from build123d import *

# Parameters (mm, degrees)
F0_W     = 24
F0_H     = 63
F1_DEPTH = 12.5
F2_W     = 3.2
F2_H     = 55
F3_DEPTH = 4
F4_W     = 16
F4_H     = 3.2
F5_DEPTH = 4


with BuildPart() as f1:
    # F0 (on Top) → F1 (new body)
    with BuildSketch(Plane.XY):
        with Locations((12, 31.5)):
            Rectangle(F0_W, F0_H)
    extrude(amount=F1_DEPTH)

    # F2 (on face) → F3 (cut)
    with BuildSketch(Plane.XY.offset(12.5)):
        with Locations((7.15, 31.5)):
            Rectangle(F2_W, F2_H)
        with Locations((12.25, 31.5)):
            Rectangle(F2_W, F2_H)
        with Locations((17.35, 31.5)):
            Rectangle(F2_W, F2_H)
    extrude(amount=-F3_DEPTH, mode=Mode.SUBTRACT)

    # F4 (on face) → F5 (cut)
    with BuildSketch(Plane.XY.offset(12.5)):
        with Locations((12, 57.4)):
            Rectangle(F4_W, F4_H)
        with BuildLine():
            Line((4, 55.8), (4, 59))
            ThreePointArc((4, 59), (2.4, 57.4), (4, 55.8))
        make_face()
        with BuildLine():
            ThreePointArc((20, 55.8), (21.6, 57.4), (20, 59))
            Line((20, 59), (20, 55.8))
        make_face()
        with Locations((12, 5.6)):
            Rectangle(F4_W, F4_H)
        with BuildLine():
            ThreePointArc((4, 7.2), (2.4, 5.6), (4, 4))
            Line((4, 4), (4, 7.2))
        make_face()
        with BuildLine():
            Line((20, 7.2), (20, 4))
            ThreePointArc((20, 4), (21.6, 5.6), (20, 7.2))
        make_face()
    extrude(amount=-F5_DEPTH, mode=Mode.SUBTRACT)


solid = f1.part
Can you work these out from the model? Positions are in its coordinate system, mm. A direction names the side the tool comes from. Coordinates: 2 decimals unless noted, no trailing zeros. Loops run counter-clockwise (first coordinate to the right, second up) from the corner with the lowest first, then second, coordinate; pieces in that order, holes last. Notation, with made-up numbers: (89.5, -18) - (97.5, -18) arc R19 cw to (97.5, 18) - close; hole circle Ø5 at (22.25, -36.5). An arc over 180 degrees is marked (long way). Put each result on its own line as item: value. Start each with the question number.
Item 1: Suppose I cut it at B-B (x = 14.75). Please give me the cut outline in (y, z).
Item 2: Suppose I cut it at A-A (y = 52). Please give me the cut outline in (x, z), and give its area (3 significant figures).
Item 3: Suppose I cut it at C-C (y = 5.6). Please give me the cut outline in (x, z).
Item 4: Which directions (+Z, -Z, +X, -X, +Y, -Y) give clear straight access to the entire face, cutting with the end or side of a thin tool? Please do faces 1 (the face through (21.6, 5.6, 10.5)), 2 (the face through (12, 32, 0)).
Item 5: If we mould it in two halves opening along Y, with no side actions, what happens to faces 3 (the face through (0, 31, 6)), 4 (the face through (10.65, 31, 11))? For each: +Y half, -Y half, draft (parallel to the pull), parting line (faces both ways), or undercut.
Item 6: If I drill on line 1 along X through (y, z) = (50.5, 11.25); line 2 along Y through (x, z) = (14.25, 10.5); line 3 along Z through (x, y) = (16, 39), over which ranges is the centre line in solid material (lowest first)?
Here are the results:
1. outline: (0, 0) - (63, 0) - (63, 12.5) - (59, 12.5) - (59, 8.5) - (55.8, 8.5) - (55.8, 12.5) - (7.2, 12.5) - (7.2, 8.5) - (4, 8.5) - (4, 12.5) - (0, 12.5) - close
2. outline: (0, 0) - (24, 0) - (24, 12.5) - (18.95, 12.5) - (18.95, 8.5) - (15.75, 8.5) - (15.75, 12.5) - (13.85, 12.5) - (13.85, 8.5) - (10.65, 8.5) - (10.65, 12.5) - (8.75, 12.5) - (8.75, 8.5) - (5.55, 8.5) - (5.55, 12.5) - (0, 12.5) - close
2. area: 262 mm²
3. outline: (0, 0) - (24, 0) - (24, 12.5) - (21.6, 12.5) - (21.6, 8.5) - (2.4, 8.5) - (2.4, 12.5) - (0, 12.5) - close
4. face 1: +Z
4. face 2: -Z, +X, -X, +Y, -Y
5. face 3: draft
5. face 4: undercut
6. line 1: 0 to 5.55, 8.75 to 10.65, 13.85 to 15.75, 18.95 to 24
6. line 2: 0 to 4, 7.2 to 55.8, 59 to 63
6. line 3: 0 to 8.5
